Autodesk Inventor part; units mm, degrees
ref_plane "YZ Plane" through (0, 0, 0) normal (1, 0, 0) x (0, 1, 0)
ref_plane "XZ Plane" through (0, 0, 0) normal (0, 1, 0) x (-1, 0, 0)
ref_plane "XY Plane" through (0, 0, 0) normal (0, 0, 1) x (1, 0, 0)
sketch "Sketch1" plane through (0, 0, 0) normal (0, 1, 0) x (-1, 0, 0)
  line L0 (59.6914, -40.823) -> (-60.3086, -40.823)
  line L1 (-65.3086, -35.823) -> (-65.3086, 34.177)
  line L2 (-60.3086, 39.177) -> (59.6914, 39.177)
  line L3 (64.6914, 34.177) -> (64.6914, -35.823)
  arc A0 (59.6914, -40.823) -> (64.6914, -35.823) centre (59.6914, -35.823) ccw
  arc A1 (-65.3086, -35.823) -> (-60.3086, -40.823) centre (-60.3086, -35.823) ccw
  arc A2 (64.6914, 34.177) -> (59.6914, 39.177) centre (59.6914, 34.177) ccw
  arc A3 (-60.3086, 39.177) -> (-65.3086, 34.177) centre (-60.3086, 34.177) ccw
  point P0 (0, 0)
  point P1 (64.6914, -40.823)
  point P2 (-65.3086, 39.177)
  point P3 (64.6914, 39.177)
  dimension "d0" = 80
  dimension "d1" = 130
  dimension "d2" = 5
  dimension "d3" = 5
  dimension "d4" = 5
  dimension "d5" = 5
extrude "Extrusion1" add sketch "Sketch1" along normal blind 2
sketch "Sketch2" plane through (0, 2, 0) normal (0, 1, 0) x (1, 0, 0)
  line L0 (-64.6914, 35.823) -> (-64.6914, -34.177)
  line L1 (-64.6914, 35.823) -> (-64.6914, -34.177)
  arc A0 (-64.6914, -34.177) -> (-59.6914, -39.177) centre (-59.6914, -34.177) ccw
  arc A1 (-64.6914, -34.177) -> (-59.6914, -39.177) centre (-59.6914, -34.177) ccw
  arc A2 (-59.6914, 40.823) -> (-64.6914, 35.823) centre (-59.6914, 35.823) ccw
  arc A3 (65.3086, 35.823) -> (60.3086, 40.823) centre (60.3086, 35.823) ccw
  arc A4 (65.3086, 35.823) -> (60.3086, 40.823) centre (60.3086, 35.823) ccw
  line L2 (-62.1914, 35.823) -> (-62.1914, -34.177)
  line L3 (65.3086, -34.177) -> (65.3086, 35.823)
  line L4 (65.3086, 35.823) -> (65.3086, -34.177)
  arc A5 (60.3086, -39.177) -> (65.3086, -34.177) centre (60.3086, -34.177) ccw
  line L5 (-59.6914, -39.177) -> (60.3086, -39.177)
  line L6 (60.3086, -39.177) -> (-59.6914, -39.177)
  line L7 (60.3086, 40.823) -> (-59.6914, 40.823)
  line L8 (-59.6914, 40.823) -> (60.3086, 40.823)
  line L9 (62.8086, 35.823) -> (62.8086, -34.177)
  line L10 (60.3086, -36.677) -> (-59.6914, -36.677)
  line L11 (-59.6914, 38.323) -> (60.3086, 38.323)
  arc A6 (-59.6914, 38.323) -> (-62.1914, 35.823) centre (-59.6914, 35.823) ccw
  arc A7 (62.8086, 35.823) -> (60.3086, 38.323) centre (60.3086, 35.823) ccw
  arc A8 (60.3086, -36.677) -> (62.8086, -34.177) centre (60.3086, -34.177) ccw
  arc A9 (-62.1914, -34.177) -> (-59.6914, -36.677) centre (-59.6914, -34.177) ccw
  arc A10 (-59.6914, 39.323) -> (-63.1914, 35.823) centre (-59.6914, 35.823) ccw
  arc A11 (63.8086, 35.823) -> (60.3086, 39.323) centre (60.3086, 35.823) ccw
  arc A12 (60.3086, -37.677) -> (63.8086, -34.177) centre (60.3086, -34.177) ccw
  arc A13 (-63.1914, -34.177) -> (-59.6914, -37.677) centre (-59.6914, -34.177) ccw
  line L12 (-63.1914, 35.823) -> (-63.1914, -34.177)
  line L13 (-59.6914, -37.677) -> (60.3086, -37.677)
  line L14 (63.8086, -34.177) -> (63.8086, 35.823)
  line L15 (60.3086, 39.323) -> (-59.6914, 39.323)
  line L16 (-59.6914, 32.323) -> (-62.1914, 32.323)
  line L17 (-56.1914, 35.823) -> (-56.1914, 38.323)
  arc A14 (-59.6914, 32.323) -> (-56.1914, 35.823) centre (-59.6914, 35.823) ccw
  line L18 (0.3086, 40.823) -> (0.3086, 33.323)
  line L19 (65.3086, 0.823) -> (44.6486, 0.823)
  line L20 (60.3086, 32.323) -> (62.8086, 32.323)
  line L21 (56.8086, 35.823) -> (56.8086, 38.323)
  arc A15 (56.8086, 35.823) -> (60.3086, 32.323) centre (60.3086, 35.823) ccw
  line L22 (-59.6914, -30.677) -> (-62.1914, -30.677)
  line L23 (-56.1914, -34.177) -> (-56.1914, -36.677)
  arc A16 (-56.1914, -34.177) -> (-59.6914, -30.677) centre (-59.6914, -34.177) ccw
  line L24 (56.8086, -34.177) -> (56.8086, -36.677)
  arc A17 (60.3086, -30.677) -> (56.8086, -34.177) centre (60.3086, -34.177) ccw
  line L25 (60.3086, -30.677) -> (62.8086, -30.677)
  point P0 (0, 0)
  point P1 (60.3086, -34.2192)
  point P2 (65.3086, -34.2192)
  point P3 (59.6599, -39.177)
  point P4 (56.8086, 38.323)
  point P5 (62.8086, -30.677)
  point P6 (56.8086, -36.677)
  point P7 (-56.1914, -36.677)
  point P8 (-62.1914, -30.677)
  dimension "d51" = 5
  dimension "d8" = 2.5
  dimension "d9" = 2.5
  dimension "d10" = 2.5
  dimension "d11" = 2.5
  dimension "d12" = 7
  dimension "d13" = 7
  dimension "d14" = 7
  dimension "d15" = 7
  dimension "d34" = 3.5
  dimension "d50" = 2.5
  dimension "d52" = 5
  dimension "d53" = 2.5
extrude "Extrusion2" add sketch "Sketch2" along normal blind 5 contours A2 L7 L18 L15 A10 L12 A13 L13 A12 L14 L19 L3 A5 L5 A0 L0 | L7 A3 L3 L19 L14 A11 L15 L18 | L17 A14 L16 L2 A6 L11 | L11 A7 L9 L20 A15 L21 | L9 A8 L10 L24 A17 L25 | L22 A16 L23 L10 A9 L2
extrude "Extrusion3" add sketch "Sketch2" along normal blind 6 contours L18 L11 A6 L2 A9 L10 A8 L9 L19 L14 A12 L13 A13 L12 A10 L15 | L15 A11 L14 L19 L9 A7 L11 L18 | L17 A14 L16 L2 A6 L11 | L11 A7 L9 L20 A15 L21 | L9 A8 L10 L24 A17 L25 | L22 A16 L23 L10 A9 L2
sketch "Sketch3" plane through (0, 0, 0) normal (0, -1, 0) x (1, 0, 0)
  circle A0 centre (60.3086, 34.177) radius 3
  line L0 (-59.6914, 39.177) -> (60.3086, 39.177)
  line L1 (65.3086, 34.177) -> (65.3086, -35.823)
  line L2 (65.3086, 24.0261) -> (65.3086, 17.2129)
  line L3 (38.477, 39.177) -> (29.3328, 39.177)
  line L4 (-59.6914, 39.177) -> (60.3086, 39.177)
  circle A1 centre (60.3086, -35.823) radius 3
  circle A2 centre (-59.6914, 34.177) radius 3
  circle A3 centre (-59.6914, -35.823) radius 3
  line L5 (-64.6914, -35.823) -> (-64.6914, 34.177)
  line L6 (60.3086, -40.823) -> (-59.6914, -40.823)
  point P0 (0, 0)
  point P1 (33.602, 39.1426)
  point P2 (55.3086, 34.177)
  point P3 (65.3086, -35.823)
  dimension "d20" = 6
  dimension "d21" = 5
  dimension "d26" = 70
  dimension "d29" = 120
  dimension "d54" = 130
  dimension "d55" = 80
  dimension "d56" = 5
extrude "Extrusion4" cut sketch "Sketch3" against normal blind 3
sketch "Sketch4" plane through (60.3086, 3, -35.823) normal (0, -1, 0) x (1, 0, 0)
  circle A0 centre (0, 0) radius 3
  point P0 (-60.3086, 35.823)
hole "Hole1" at (60.3086, 3, -35.823) direction (0, 1, 0) diameter 3.5 end through all
pattern_linear "Rectangular Pattern1" count 2 spacing 120 along (-1, 0, 0) count 2 spacing 70 along (0, 0, 1) of "Hole1"
sketch "Sketch6" plane through (0, 2, 0) normal (0, 1, 0) x (1, 0, 0)
  circle A0 centre (50.3086, -29.177) radius 3.5
  line L0 (65.3086, -34.177) -> (65.3086, 35.823)
  line L1 (-59.6914, -39.177) -> (60.3086, -39.177)
  line L2 (65.3086, -34.177) -> (65.3086, 35.823)
  line L3 (65.3086, -6.9039) -> (65.3086, -1.4927)
  line L4 (16.8866, -39.177) -> (12.0352, -39.177)
  circle A1 centre (50.3086, -29.177) radius 1.97
  point P0 (0, 0)
  dimension "d57" = 7
  dimension "d58" = 15
  dimension "d59" = 10
  dimension "d60" = 3.94
extrude "Extrusion5" add sketch "Sketch6" along normal blind 6
pattern_linear "Rectangular Pattern2" count 2 spacing 53 along (0, 0, -1) count 2 spacing 100 along (-1, 0, 0) of "Extrusion5"
sketch "Sketch7" plane through (0, 2, 0) normal (0, 1, 0) x (1, 0, 0)
  circle A0 centre (25.3086, -24.177) radius 4.5
  line L0 (-59.6914, -39.177) -> (60.3086, -39.177)
  line L1 (65.3086, -34.177) -> (65.3086, 35.823)
  circle A1 centre (25.3086, -24.177) radius 2.175
  point P0 (0, 0)
  dimension "d69" = 9
  dimension "d70" = 15
  dimension "d71" = 40
  dimension "d72" = 4.35
extrude "Extrusion6" add sketch "Sketch7" along normal blind 4
sketch "Sketch8" plane through (25.3086, 2, 24.177) normal (0, 1, 0) x (1, 0, 0)
  circle A0 centre (0, 0) radius 2.175
  point P0 (-25.3086, 24.177)
hole "Hole2" at (25.3086, 2, 24.177) direction (0, -1, 0) diameter 4.35 end through all
pattern_linear "Rectangular Pattern4" count 2 spacing 50 along (-1, 0, 0) count 2 spacing 50 along (0, 0, -1) of "Extrusion6", "Hole2"
chamfer "Chamfer1" distance 1 angle 45 8 edges at (0.3086, 0, 39.177) (63.8442, 0, 37.7125) (65.3086, 0, -0.823) (63.8442, 0, -39.3586) (0.3086, 0, -40.823) (-63.2269, 0, -39.3586) (-64.6914, 0, -0.823) (-63.2269, 0, 37.7125)
sketch "Sketch9" plane through (0, 2, 0) normal (0, 1, 0) x (1, 0, 0)
  line L0 (46.8086, 34.323) -> (-3.1914, 34.323)
  line L1 (-3.1914, 34.323) -> (-3.1914, 36.323)
  line L2 (-3.1914, 36.323) -> (46.8086, 36.323)
  line L3 (46.8086, 36.323) -> (46.8086, 34.323)
  line L4 (-56.1914, 38.323) -> (56.8086, 38.323)
  line L5 (56.8086, 38.323) -> (56.8086, 35.823)
  line L6 (-3.1914, 38.323) -> (46.8086, 38.323)
  line L7 (46.8086, 38.323) -> (46.8086, 37.323)
  line L8 (-3.1914, 37.323) -> (-3.1914, 38.323)
  point P0 (0, 0)
  point P1 (46.8086, 35.323)
  dimension "d97" = 50
  dimension "d98" = 2
  dimension "d99" = 2
  dimension "d100" = 10
  dimension "d103" = 50
extrude "Extrusion7" add sketch "Sketch9" along normal blind 4
equation "\"d3\" = d2"
equation "\"d4\" = d2"
equation "\"d5\" = d2"
equation "\"d9\" = d8"
equation "\"d10\" = d8"
equation "\"d11\" = d8"
equation "\"d52\" = d51"
equation "\"d53\" = d50"
equation "\"d103\" = d97"
properties part number "housing_bottom"
Can you work these out from the model? Positions are in its coordinate system, mm. A direction names the side the tool comes from. Coordinates: 2 decimals unless noted, no trailing zeros. Write each loop counter-clockwise with the first axis right and the second up, starting at its lowest first coordinate (ties: lowest second). Pieces come first, ordered by that corner, then holes. Notation, with made-up numbers: M 20.5,68 L 62.5,68 A32 ccw 62.5,103 Z; hole C 0,77 d8. An arc over 180 degrees is marked long. Write item = value, one per line. Start each with the question number.
Q1. Thinking about a two-plate mould opening in Z: for faces 1 (the face through (1, 0, 0)), 2 (the face through (-58, 3, 33)), 3 (the face through (63.883, 3.958, 37.673)), 4 (the face through (56.809, 5, -37)), which applies, released by +Z, released by -Z, zero draft, split by the parting line, or undercut?
Q2. I'm going to push flat-ended pins straight in: pin 1 (0.5 mm diameter, centred on x = 25, y = 7.5, fed in from -Z); pin 2 (5.5 mm diameter, centred on x = 60.31, z = 34.18, fed in from -Y); pin 3 (2 mm diameter, centred on y = 6, z = -37, fed in from -X). Where does each tip first touch, or does it pass through?
Q3. On a 3-axis mill with a long thin cutter (end or side, diameter ignored), from which of +Z, -Z, +X, -X, +Y, -Y can I reach the whole of each face in a straight line? I mean faces 5 (the face through (1, 4, 39.177)), 6 (the face through (-50, 2, 29)), 7 (the face through (62, 3, -37)). Say none if no direction works.
Q4. If we section it at A-A, the plane x = -18.5: Write out the boundary of the cut face in (y, z), then the cut area to 3 significant figures.
Q5. If I drill on L1, parallel to Z at x = 5.5, y = 4.5; L2, parallel to X at y = 6.75, z = -35.5; L3, parallel to Z at x = -30, y = 4, over which ranges is the centre line in solid material (lowest first)? Write a range as [from, to].
Q6. If we section it at B-B, the plane x = 35: Write out the boundary of the cut face in (y, z), then the cut area to 3 significant figures.
Check sheet entries:
q1.face_1 = zero draft
q1.face_2 = undercut
q1.face_3 = released by +Z
q1.face_4 = undercut
q2.pin_1 = -39.32
q2.pin_2 = 3
q2.pin_3 = -64.69
q3.face_5 = +Z, +X, -X, +Y, -Y
q3.face_6 = +Y
q3.face_7 = -Y
q4.outline = M 0,-39.82 L 1,-40.82 L 7,-40.82 L 7,-39.32 L 8,-39.32 L 8,-38.32 L 2,-38.32 L 2,36.68 L 8,36.68 L 8,37.68 L 7,37.68 L 7,39.18 L 1,39.18 L 0,38.18 Z
q4.area = 186 mm²
q5.L1 = [-40.82, -38.32], [-36.32, -34.32], [36.68, 39.18]
q5.L2 = [-64.69, -61.41], [-57.97, -56.21], [56.82, 58.59], [62.03, 65.31]
q5.L3 = [-40.82, -38.32], [36.68, 39.18]
q6.outline = M 0,-39.82 L 1,-40.82 L 7,-40.82 L 7,-39.32 L 8,-39.32 L 8,-38.32 L 2,-38.32 L 2,-36.32 L 6,-36.32 L 6,-34.32 L 2,-34.32 L 2,36.68 L 8,36.68 L 8,37.68 L 7,37.68 L 7,39.18 L 1,39.18 L 0,38.18 Z
q6.area = 194 mm²
